Autodesk Inventor part; units mm, degrees
ref_plane "Start plane" through (0, 0, -19.05) normal (0, 0, 1) x (1, 0, 0)
ref_plane "End plane" through (0, 0, 660.4) normal (0, 0, 1) x (1, 0, 0)
ref_plane "Work Plane4" through (0, 19.05, 660.4) normal (0, -0.7071, 0.7071) x (1, 0, 0)
ref_plane "Start plane" through (0, 0, -19.05) normal (0, 0, 1) x (1, 0, 0)
ref_plane "End plane" through (0, 0, 660.4) normal (0, 0, 1) x (1, 0, 0)
sketch "Sketch" plane through (0, 0, 0) normal (0, 0, 1) x (1, 0, 0)
  circle A0 centre (0, 0) radius 19.05
  dimension "d0" = 38.1
extrude "Body" add sketch "Sketch" along normal up to surface (679.45 mm away) from surface at -19.05
sketch "Sketch2" plane through (0, 0, 0) normal (0, 0, 1) x (1, 0, 0)
  line L0 (0, 0) -> (10, 0)
ref_plane "Work Plane3" through (0, 0, 0) normal (0, -1, 0) x (1, 0, 0)
sketch "Sketch3" plane through (0, 0, 0) normal (0, -1, 0) x (1, 0, 0)
  line L0 (-2, -19.05) -> (12, -19.05)
  line L1 (-2, 660.4) -> (12, 660.4)
  dimension "d7" = 679.45
ref_plane "Work Plane4" through (0, 19.05, 660.4) normal (0, -0.7071, 0.7071) x (1, 0, 0)
split "Split1" plane through (0, 19.05, 660.4) removes the side toward (0, -0.7071, 0.7071)
ref_plane "Work Plane5" through (0, 19.05, -19.05) normal (0, -0.7071, -0.7071) x (1, 0, 0)
split "Split2" plane through (0, 19.05, -19.05) removes the side toward (0, -0.7071, -0.7071)
equation "\"d0\" = Diam"
equation "\"d1\" = G_L"
equation "\"Diam\" = 38.1"
equation "\"G_L\" = d7"
equation "\"G_OFFSET_START\" = 19.05"
equation "\"G_OFFSET_END\" = 19.05"
equation "\"d4\" = -G_OFFSET_START"
equation "\"d5\" = G_OFFSET_END + B_L"
equation "\"B_L\" = 641.35"
properties part number "ANSI/AISC Rolled Steel - 1 1/2-26.75" material "Steel, Mild"
The listing builds one solid part. Answer for the finished solid, in the listing's coordinates (mm). Coordinates: 2 decimals unless noted, no trailing zeros. Loops run counter-clockwise (first coordinate to the right, second up) from the corner with the lowest first, then second, coordinate; pieces in that order, holes last. Notation, with made-up numbers: (64, -20) -> (70, -20) arc R25 ccw to (70, 3) -> close; hole circle Ø11 at (62.5, 45). An arc over 180 degrees is marked (long way). Answer in a Markdown table with one row per item. Add a question column.
1. The part is cut by section C-C, the plane y = 0. Write down the section's boundary in (x, z), then the cut area to 3 significant figures.
2. Flat-ended cylindrical pins translate along their axes: P1, Ø8, axis at x = -8, y = -10, coming from the -Z side; P2, Ø2, axis at x = -13, y = -2.5, coming from the +Z side; P3, Ø3, axis at x = -8, z = 275.5, coming from the +Y side; P4, Ø1, axis at y = -0.5, z = 417.5, coming from the +X side. Find the tip coordinate at first contact, or state that the pin passes through.
3. The part is cut by section A-A, the plane x = 0. Write down the section's boundary in (y, z), then the cut area to 3 significant figures.
4. The part is cut by section B-B, the plane z = 168. Write down the section's boundary in (x, y), then the cut area to 3 significant figures.
5. Consider line 1 (X direction, y = -1, z = 266); line 2 (X direction, y = 2, z = 258.5). Determine where each line is inside the solid, lowest interval first. Write a range as [from, to].
Answer below:
| question | item | result |
|---|---|---|
| 1 | outline | (-19.05, 0) -> (19.05, 0) -> (19.05, 641.35) -> (-19.05, 641.35) -> close |
| 1 | area | 24,400 mm2 |
| 2 | P1 | z = 6 |
| 2 | P2 | z = 639.85 |
| 2 | P3 | y = 17.91 |
| 2 | P4 | x = 19.05 |
| 3 | outline | (-19.05, 19.05) -> (19.05, -19.05) -> (19.05, 660.4) -> (-19.05, 622.3) -> close |
| 3 | area | 24,400 mm2 |
| 4 | outline | circle Ø38.1 at (0, 0) |
| 4 | area | 1,140 mm2 |
| 5 | line 1 | [-19.02, 19.02] |
| 5 | line 2 | [-18.94, 18.94] |
